Could you check a few things on this drawing? It's one solid part, dimensions in mm from its lowest x, y, z. Coordinates: 2 decimals unless noted, no trailing zeros. Write each loop counter-clockwise with the first axis right and the second up, starting at its lowest first coordinate (ties: lowest second). Pieces come first, ordered by that corner, then holes. Notation, with made-up numbers: (27, 73) - (52, 73) arc R22 ccw to (52, 80) - close; hole circle Ø9 at (23.25, -27). An arc over 180 degrees is marked (long way). Write item = value, one per line. Start each with the question number.
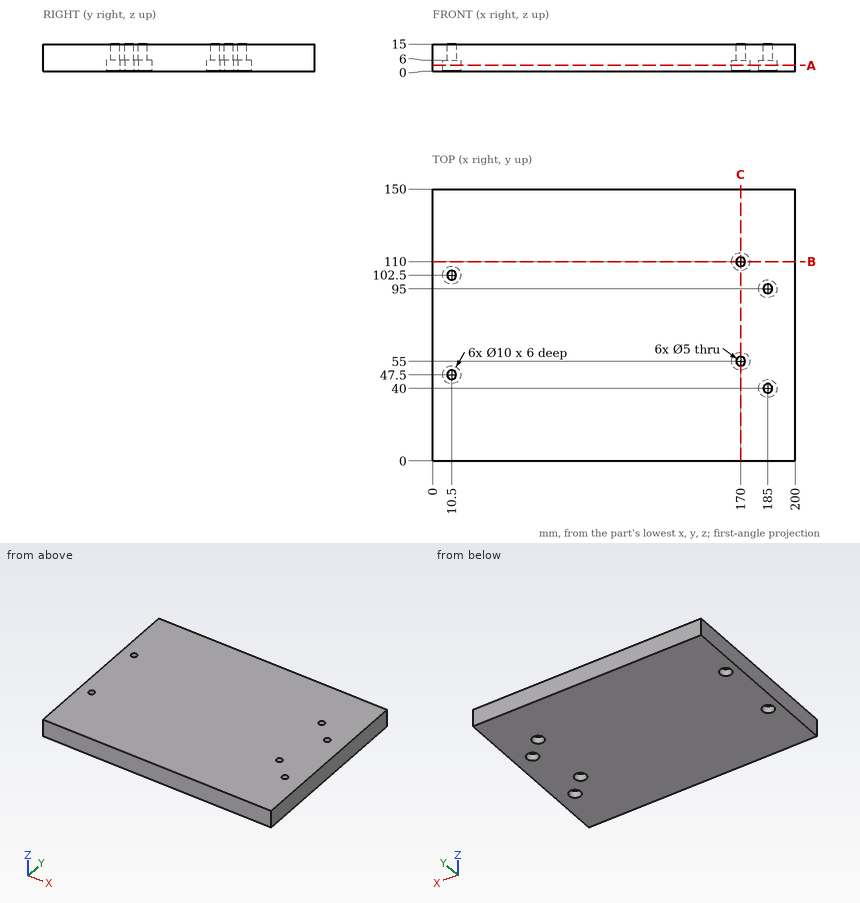
1) Suppose I cut it at B-B on y = 110. Please give me the cut outline in (x, z).
2) Suppose I cut it at A-A on z = 3.25. Please give me the cut outline in (x, y), plus the area to 3 significant figures.
3) If I drill on probe 1 along Y at (x, z) = (10.5, 12.75); probe 2 along Y at (x, z) = (170, 4.1); probe 3 along X at (y, z) = (94, 8), over which ranges is the centre line in solid material (lowest first)? Write a range as [from, to].
4) Suppose I cut it at C-C on x = 170. Please give me the cut outline in (y, z).
5) For P1, Ø4, axis at x = 185, y = 95, coming from the +Z side; P2, Ø3, axis at x = 185.5, y = 42.5, coming from the -Z side, each with a flat end and sliding along its axis, tell me the tip position at first contact or that it passes through.
Reply:
q1.outline = (0, 0) - (165, 0) - (165, 6) - (167.5, 6) - (167.5, 15) - (0, 15) - close; (172.5, 6) - (175, 6) - (175, 0) - (200, 0) - (200, 15) - (172.5, 15) - close
q2.outline = (0, 0) - (200, 0) - (200, 150) - (0, 150) - close; hole circle Ø10 at (10.5, 47.5); hole circle Ø10 at (10.5, 102.5); hole circle Ø10 at (170, 55); hole circle Ø10 at (170, 110); hole circle Ø10 at (185, 40); hole circle Ø10 at (185, 95)
q2.area = 29,500 mm^2
q3.probe_1 = [0, 45], [50, 100], [105, 150]
q3.probe_2 = [0, 50], [60, 105], [115, 150]
q3.probe_3 = [0, 182.71], [187.29, 200]
q4.outline = (0, 0) - (50, 0) - (50, 6) - (52.5, 6) - (52.5, 15) - (0, 15) - close; (57.5, 6) - (60, 6) - (60, 0) - (105, 0) - (105, 6) - (107.5, 6) - (107.5, 15) - (57.5, 15) - close; (112.5, 6) - (115, 6) - (115, 0) - (150, 0) - (150, 15) - (112.5, 15) - close
q5.P1 = through
q5.P2 = 6
